```python
from build123d import *

# Parameters (mm, degrees)
BASPROSKE_W                   = 10
BASPROSKE_H                   = 11
TOOTHCUT_DEPTH                = 19.493242009
TEETHCUTS_COUNT               = 20
TEETHCUTS_ANGLE               = 342
BORSKE_R                      = 0.4
BORE_DEPTH                    = 50.0000508
TALADRO_DE_MARGEN_PARA_M101_D = 10.5
CROQUIS3_R                    = 5.25
CROQUIS3_R_2                  = 2.5
SALIENTE_EXTRUIR1_DEPTH       = 5


with BuildPart() as part:
    # BasProSke → Base-Revolve (revolve)
    with BuildSketch(Plane(origin=(0, 0, 0), x_dir=(1, 0, 0), z_dir=(0, 1, 0)), mode=Mode.PRIVATE) as base_revolve_sk:
        with Locations((5, 5.5)):
            Rectangle(BASPROSKE_W, BASPROSKE_H)
    revolve(base_revolve_sk.sketch.rotate(Axis((-10, 0, 0), (1, 0, 0)), 180), axis=Axis((-10, 0, 0), (1, 0, 0)))

    # TooCutSke → ToothCut (cut, through all)
    with BuildSketch(Plane(origin=(0, 0, 0), x_dir=(0, 0, -1), z_dir=(1, 0, 0))):
        with BuildLine():
            ThreePointArc((0.499924007, 8.734705318), (0, 8.749), (-0.499924007, 8.734705318))
            ThreePointArc((-0.499924007, 8.734705318), (-0.824302243, 9.905497836), (-1.485192705, 10.924909509))
            ThreePointArc((-1.485192705, 10.924909509), (0, 11.0254), (1.485192705, 10.924909509))
            ThreePointArc((1.485192705, 10.924909509), (0.824302243, 9.905497836), (0.499924007, 8.734705318))
        make_face()
    toothcut = extrude(amount=TOOTHCUT_DEPTH, mode=Mode.SUBTRACT)

    # TeethCuts: ToothCut ×20 about axis
    teethcuts_axis = Axis((-10, 0, 0), (1, 0, 0))
    for i in range(1, TEETHCUTS_COUNT):
        add(toothcut.rotate(teethcuts_axis, i * TEETHCUTS_ANGLE / (TEETHCUTS_COUNT - 1)), mode=Mode.SUBTRACT)

    # BorSke → Bore (cut, symmetric)
    with BuildSketch(Plane(origin=(0, 0, 0), x_dir=(0, 0, -1), z_dir=(1, 0, 0))):
        with Locations(Location((0, 0, 0), (0, 0, 180))):
            Circle(BORSKE_R)
    extrude(amount=BORE_DEPTH, both=True, mode=Mode.SUBTRACT)

    # Taladro de margen para M101 (through all)
    with Locations(Plane(origin=(10, 0, 0), x_dir=(0, 0, -1), z_dir=(1, 0, 0))):
        with Locations((0, 0)):
            Hole(TALADRO_DE_MARGEN_PARA_M101_D / 2)

    # Croquis3 → Saliente-Extruir1 (add)
    with BuildSketch(Plane.ZY):
        with Locations(Location((0, 0, 0), (0, 0, 180))):
            Circle(CROQUIS3_R)
        Circle(CROQUIS3_R_2, mode=Mode.SUBTRACT)
    extrude(amount=-SALIENTE_EXTRUIR1_DEPTH)


solid = part.part
```
Geometry check sheet. Reference: the model listing, model coordinates, mm. A direction names the side the tool comes from. Give positions to 0.01 mm unless a question says otherwise; leave off trailing zeros. Loops run counter-clockwise (first coordinate to the right, second up) from the corner with the lowest first, then second, coordinate; pieces in that order, holes last. Notation, with made-up numbers: M 5.25,51.25 L 51.25,51.25 A28 ccw 51.25,88.25 Z; hole C 71,3.5 d9. An arc over 180 degrees is marked long. Write item = value, one per line. Start each with the question number.
1. Thickness scan on probe 1 along Z at (x, y) = (6.45, 0); probe 2 along Y at (x, z) = (5, -9). Record the ranges inside material, lowest first.
2. Section check A-A, the plane y = 0. Enter the section's corners in (x, z).
3. Tool access check on faces 5 (the face through (7.5, 1.6, 5)), 6 (the face through (4.93, -6.461, 7.513)), 7 (the face through (4.93, 9.677, 2.277)), 8 (the face through (4.93, -0.825, -9.907)). Record the directions out of +Z, -Z, +X, -X, +Y, -Y that give a thin tool (end or side, any length) a straight path to the whole face; none if there is none.
4. Go/stop test with flat-tipped pins: P1, Ø4, axis at x = 6.5, y = -4.5, coming from the +Z side; P2, Ø3, axis at y = 0, z = 0.5, coming from the +X side; P3, Ø4, axis at x = 3, z = -8, coming from the +Y side. Record where each tip stops, or that it passes through.
5. Draft check along Y on faces 1 (the face through (4.93, -8.75, 0.01)), 2 (the face through (4.93, -2.28, -9.64)), 3 (the face through (0, 2, -2)), 4 (the face through (4.93, 8.75, -0.01)). Enter one of: +Y half, -Y half, draft (parallel to the pull), parting line (faces both ways), or undercut.
Values follow:
q1.probe_1 = -8.75 to -5.25, 5.25 to 8.75
q1.probe_2 = -5.23 to -3.7, -2.29 to -0.54, 0.54 to 2.29, 3.7 to 5.23
q2.outline = M 0,-8.75 L 10,-8.75 L 10,-5.25 L 5,-5.25 L 5,-2.5 L 0,-2.5 Z; M 0,2.5 L 5,2.5 L 5,5.25 L 10,5.25 L 10,8.75 L 0,8.75 Z
q3.face_5 = +X
q3.face_6 = +Z, +X, -X
q3.face_7 = +X, -X
q3.face_8 = -Z, +X, -X
q4.P1 = 9.92
q4.P2 = through
q4.P3 = 7.96
q5.face_1 = -Y half
q5.face_2 = undercut
q5.face_3 = draft
q5.face_4 = +Y half
